from build123d import *

# Parameters (mm, degrees)
SKETCH1_W                 = 38.1
SKETCH1_H                 = 31.75
BOSS_EXTRUDE1_DEPTH       = 9.525
F_6_32_TAPPED_HOLE1_D     = 2.7051
F_6_32_TAPPED_HOLE1_DEPTH = 7.62
F_6_32_TAPPED_HOLE1_TIP   = 0.81269403
F_6_32_TAPPED_HOLE2_D     = 2.7051
F_6_32_TAPPED_HOLE2_DEPTH = 9.38784
F_6_32_TAPPED_HOLE2_TIP   = 0.81269403
SKETCH2_R                 = 2.54
CUT_EXTRUDE1_DEPTH        = 39.232062788


with BuildPart() as part:
    # Sketch1 → Boss-Extrude1 (new body)
    with BuildSketch(Plane.XY):
        Rectangle(SKETCH1_W, SKETCH1_H)
    extrude(amount=BOSS_EXTRUDE1_DEPTH)

    # #6-32 Tapped Hole1
    with Locations(Plane(origin=(0, 15.875, 0), x_dir=(1, 0, 0), z_dir=(0, 1, 0))):
        with Locations((-14.2875, -4.7625), (14.2875, -4.7625)):
            Hole(F_6_32_TAPPED_HOLE1_D / 2, depth=F_6_32_TAPPED_HOLE1_DEPTH)
            with Locations((0, 0, -(F_6_32_TAPPED_HOLE1_DEPTH + F_6_32_TAPPED_HOLE1_TIP / 2))):  # 118° drill point
                Cone(0, F_6_32_TAPPED_HOLE1_D / 2, F_6_32_TAPPED_HOLE1_TIP, mode=Mode.SUBTRACT)

    # #6-32 Tapped Hole2
    with Locations(Plane(origin=(0, -15.875, 0), x_dir=(-1, 0, 0), z_dir=(0, -1, 0))):
        with Locations((-14.2875, -4.7625), (14.2875, -4.7625)):
            Hole(F_6_32_TAPPED_HOLE2_D / 2, depth=F_6_32_TAPPED_HOLE2_DEPTH)
            with Locations((0, 0, -(F_6_32_TAPPED_HOLE2_DEPTH + F_6_32_TAPPED_HOLE2_TIP / 2))):  # 118° drill point
                Cone(0, F_6_32_TAPPED_HOLE2_D / 2, F_6_32_TAPPED_HOLE2_TIP, mode=Mode.SUBTRACT)

    # Sketch2 → Cut-Extrude1 (cut, through all)
    with BuildSketch(Plane(origin=(0, 15.875, 0), x_dir=(1, 0, 0), z_dir=(0, 1, 0))):
        with Locations(Location((-14.2875, -4.7625, 0), (0, 0, 270))):
            Circle(SKETCH2_R)
        with Locations(Location((14.2875, -4.7625, 0), (0, 0, 270))):
            Circle(SKETCH2_R)
    extrude(amount=-CUT_EXTRUDE1_DEPTH, mode=Mode.SUBTRACT)


solid = part.part
For this review, take the finished solid that the model builds, in its own axes (mm). Give positions to 0.01 mm unless a question says otherwise; leave off trailing zeros. Loops run counter-clockwise (first coordinate to the right, second up) from the corner with the lowest first, then second, coordinate; pieces in that order, holes last. Notation, with made-up numbers: M 36.25,-2 L 69.25,-2 A15 ccw 69.25,2 Z; hole C 33,-33.75 d5. An arc over 180 degrees is marked long. Answer as a JSON object with one key per item and string values. Group by question number.
Q1. Add section A-A on z = 6.5. Give the boundary of the cut face in (x, y) (3 decimals).
Q2. For probe 1 along Z at (x, y) = (14.5, 2) (3 decimals); probe 2 along X at (y, z) = (-1.5, 5.5); probe 3 along X at (y, z) = (-13.5, 2.75), list the stretches that pass through material, from the lowest coordinate up. Write a range as [from, to].
Q3. Add section B-B on y = -14. Give the number of separate pieces and of enclosed holes in the cut face, and give its area (3 significant figures).
Q4. Mouldability with a two-part tool opening along X and no side actions: class faces 1 (the flat face through (19.05, 0, 5)), 2 (the flat face through (0, -15.875, 5)), 3 (the cylindrical face through (-16.767, 0.222, 4.212)), 4 (the flat face through (-19.05, 0, 5)) as +X half, -X half, draft (parallel to the pull), parting line (faces both ways), or undercut.
Q5. Insertion check: P1, Ø4, axis at x = -14.29, z = 4.76, coming from the -Y side. The pin has a flat end and moves straight along its axis. Give the tip position at first contact, or say it passes through.
Q6. Add section C-C on z = 2.75. Give the boundary of the cut face in (x, y) (3 decimals).
Checked values:
{
 "1": {"outline": "M -19.05,-15.875 L -16.14,-15.875 L -16.14,15.875 L -19.05,15.875 Z; M -12.435,-15.875 L 12.435,-15.875 L 12.435,15.875 L -12.435,15.875 Z; M 16.14,-15.875 L 19.05,-15.875 L 19.05,15.875 L 16.14,15.875 Z"},
 "2": {"probe 1": "[0, 2.231], [7.294, 9.525]", "probe 2": "[-19.05, -16.72], [-11.86, 11.86], [16.72, 19.05]", "probe 3": "[-19.05, -15.84], [-12.74, 12.74], [15.84, 19.05]"},
 "3": {"separate pieces": "1", "enclosed holes": "2", "area": "322 mm²"},
 "4": {"face 1": "+X half", "face 2": "draft", "face 3": "undercut", "face 4": "-X half"},
 "5": {"P1": "through"},
 "6": {"outline": "M -19.05,-15.875 L -15.837,-15.875 L -15.837,15.875 L -19.05,15.875 Z; M -12.738,-15.875 L 12.738,-15.875 L 12.738,15.875 L -12.738,15.875 Z; M 15.837,-15.875 L 19.05,-15.875 L 19.05,15.875 L 15.837,15.875 Z"}
}
